Source: three-view drawing plus pictorial views. Frame: mm from the lowest corner of the part. A direction names the side the tool comes from. Give positions to 0.01 mm unless a question says otherwise; leave off trailing zeros. Loops run counter-clockwise (first coordinate to the right, second up) from the corner with the lowest first, then second, coordinate; pieces in that order, holes last.
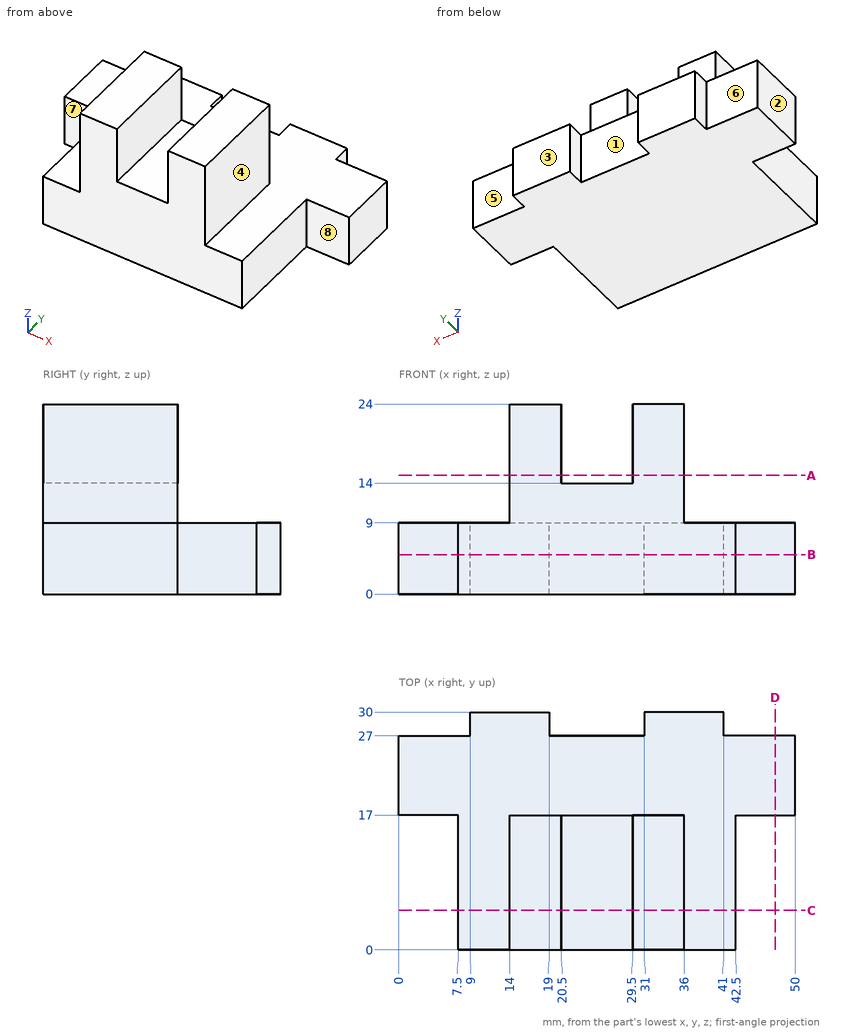
(1) Cut plane C-C (y = 5). Return the cut outline in (x, z).
Values follow:
outline: (7.5, 0) - (42.5, 0) - (42.5, 9) - (36, 9) - (36, 24) - (29.5, 24) - (29.5, 14) - (20.5, 14) - (20.5, 24) - (14, 24) - (14, 9) - (7.5, 9) - close
(2) Cut plane A-A (z = 15). Return the cut outline in (x, y).
Values follow:
outline: (14, 0) - (20.5, 0) - (20.5, 17) - (14, 17) - close; (29.5, 0) - (36, 0) - (36, 17) - (29.5, 17) - close
(3) Pin query (flat end, axial travel): pin 1 Ø7 at (x, z) = (25.5, 5) entering from +Y; pin 2 Ø4 at (x, z) = (5, 2.5) entering from -Y; pin 3 Ø2.5 at (y, z) = (28.5, 2.5) entering from -X; pin 4 Ø1.5 at (x, y) = (40.5, 13) entering from -Z. Return the tip coordinate at first contact, or that it passes through.
Values follow:
pin 1: stops at y = 27
pin 2: stops at y = 17
pin 3: stops at x = 9
pin 4: stops at z = 0
(4) Cut plane B-B (z = 5). Return the cut outline in (x, y), and give its area (4 significant figures).
Values follow:
outline: (0, 17) - (7.5, 17) - (7.5, 0) - (42.5, 0) - (42.5, 17) - (50, 17) - (50, 27) - (41, 27) - (41, 30) - (31, 30) - (31, 27) - (19, 27) - (19, 30) - (9, 30) - (9, 27) - (0, 27) - close
area: 1,155 mm2
(5) Mould query, pull axis X, two halves, no side actions, for the marked faces 1, 2, 3 and 4. Classes: +X half, -X half, draft (parallel to the pull), parting line (faces both ways), or undercut.
Values follow:
face 1: undercut
face 2: -X half
face 3: draft
face 4: +X half
(6) Ray query, probe 1 along X at (y, z) = (11.5, 17.25); probe 2 along X at (y, z) = (28.5, 6.5); probe 3 along X at (y, z) = (7, 13.5). Return the intervals inside material, ascending.
Values follow:
probe 1: x = 14 to 20.5, 29.5 to 36
probe 2: x = 9 to 19, 31 to 41
probe 3: x = 14 to 36
(7) Cut plane D-D (x = 47.5). Return the cut outline in (y, z).
Values follow:
outline: (17, 0) - (27, 0) - (27, 9) - (17, 9) - close
(8) Reachability of the marked faces 5, 6, 7 and 8 from +Z, -Z, +X, -X, +Y, -Y: full face, straight path, thin tool, end or side. Return the list, or none.
Values follow:
face 5: +Z, -Z, +X, +Y
face 6: +Z, -Z, -X, +Y
face 7: +Z, -Z, -X, -Y
face 8: +Z, -Z, +X, -Y
